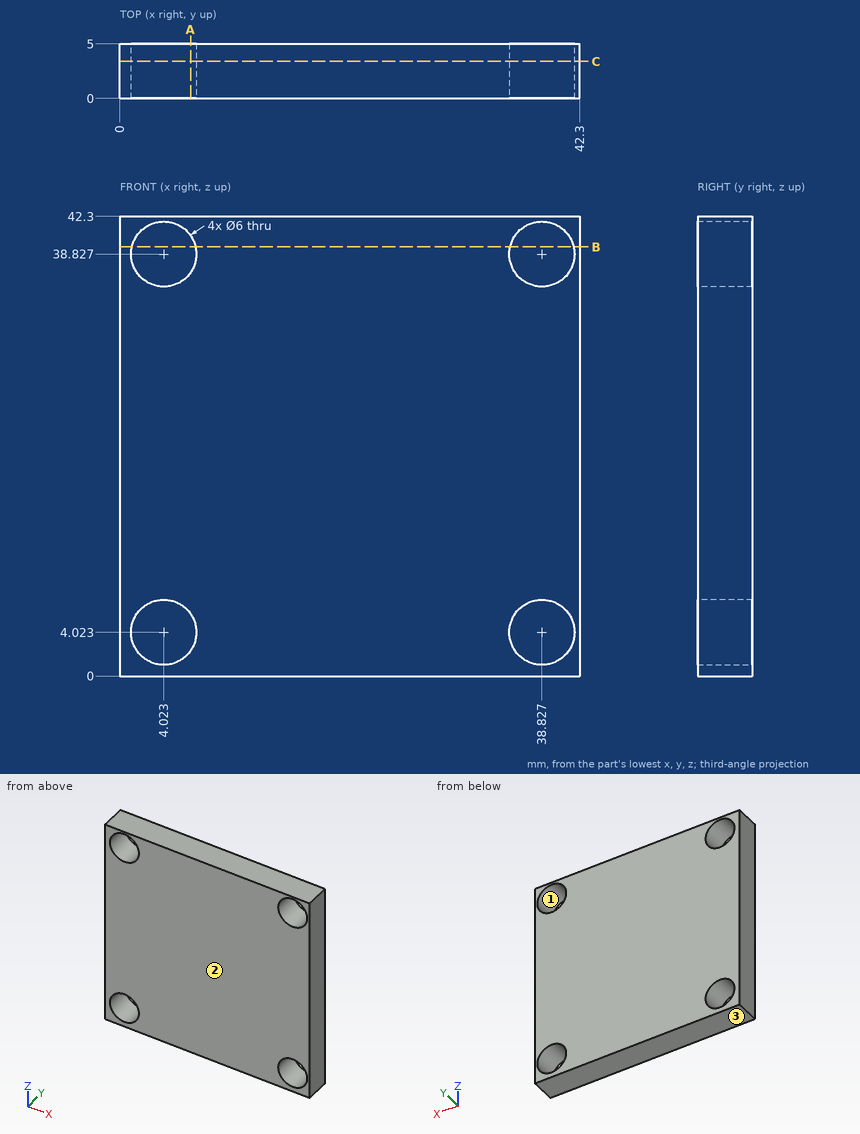
Drawing for the job (mm, zero at the part's lowest x, y, z). Coordinates: 2 decimals unless noted, no trailing zeros. Loops run counter-clockwise (first coordinate to the right, second up) from the corner with the lowest first, then second, coordinate; pieces in that order, holes last. Notation, with made-up numbers: (-2, 16.5) - (37, 16.5) arc R30 ccw to (37, 38.5) - close; hole circle Ø3 at (-29, 73.5). An arc over 180 degrees is marked (long way). Use CSV: the item, a comma, the result in double quotes. Start each with the question number.
Q1. Drop a flat-ended pin along its axis: P1, Ø10, axis at x = 26.5, z = 6, coming from the -Y side. Give the stop position or say it passes through.
Q2. Cut at C-C, the plane y = 3.4. List the corners of the cut face in (x, z), then the cut area to 3 significant figures.
Q3. Two-plate mould, pull along Z, no slides. Class the marked faces 1, 2 and 3: +Z half, -Z half, draft (parallel to the pull), parting line (faces both ways), or undercut.
Q4. Probe probe 1 along Z at (x, y) = (4, 2.9); probe 2 along Z at (x, y) = (4.5, 2.1) (1 decimal); probe 3 along X at (y, z) = (0.85, 3.5). List the from-to ranges inside material, lowest first. Write a range as from..to.
Q5. Cut at A-A, the plane x = 6.5. List the corners of the cut face in (y, z) (1 decimal), then the cut area to 3 significant figures.
Q6. Cut at B-B, the plane z = 39.5. List the corners of the cut face in (x, y).
Here are the results:
1,P1,"y = 0"
2,outline,"(0, 0) - (42.3, 0) - (42.3, 42.3) - (0, 42.3) - close; hole circle Ø6 at (4.02, 4.02); hole circle Ø6 at (4.02, 38.83); hole circle Ø6 at (38.83, 4.02); hole circle Ø6 at (38.83, 38.83)"
2,area,"1,680 mm2"
3,face 1,"undercut"
3,face 2,"draft"
3,face 3,"-Z half"
4,probe 1,"0..1.02, 7.02..35.83, 41.83..42.3"
4,probe 2,"0..1.1, 7..35.9, 41.8..42.3"
4,probe 3,"0..1.07, 6.98..35.87, 41.78..42.3"
5,outline,"(0, 0) - (5, 0) - (5, 2.3) - (0, 2.3) - close; (0, 5.7) - (5, 5.7) - (5, 37.1) - (0, 37.1) - close; (0, 40.5) - (5, 40.5) - (5, 42.3) - (0, 42.3) - close"
5,area,"178 mm2"
6,outline,"(0, 0) - (1.1, 0) - (1.1, 5) - (0, 5) - close; (6.95, 0) - (35.9, 0) - (35.9, 5) - (6.95, 5) - close; (41.75, 0) - (42.3, 0) - (42.3, 5) - (41.75, 5) - close"
